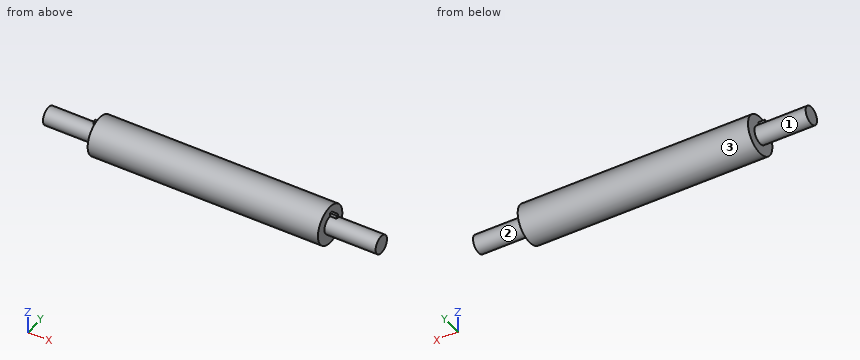
from build123d import *

# Parameters (mm, degrees)
BOSS_EXTRUDE1_START = 5
BOSS_EXTRUDE1_DEPTH = 5


with BuildPart() as part:
    # Sketch2 → Revolve1 (revolve)
    with BuildSketch(Plane.XY, mode=Mode.PRIVATE) as revolve1_sk:
        Polygon((130, 0), (-130, 0), (-130, -7), (-90, -7), (-90, -15), (90, -15), (90, -7), (130, -7), align=None)
    revolve(revolve1_sk.sketch.rotate(Axis((130, 0, 0), (-1, 0, 0)), 180), axis=Axis((130, 0, 0), (-1, 0, 0)))

    # Sketch3 → Boss-Extrude1 (add)
    with BuildSketch(Plane(origin=(90, 0, 0), x_dir=(0, 0, -1), z_dir=(1, 0, 0)).offset(BOSS_EXTRUDE1_START)):
        with BuildLine():
            Line((-7, 0), (-9.611930855, 0))
            Line((-9.611930855, 0), (-9.611930855, 2.103316634))
            Line((-9.611930855, 2.103316634), (-6.676530471, 2.103316634))
            ThreePointArc((-6.676530471, 2.103316634), (-6.918660033, 1.064022251), (-7, 0))
        make_face()
    boss_extrude1 = extrude(amount=-BOSS_EXTRUDE1_DEPTH)

    # Mirror1: Boss-Extrude1 across plane
    add(boss_extrude1.mirror(Plane(origin=(0, 0, 0), x_dir=(0, 0, 1), z_dir=(1, 0, 0))))


solid = part.part
Work out the finished part from the listing and answer in its coordinate system (mm). Face numbers are marked on the shaded views. A direction names the side the tool comes from. Coordinates: 2 decimals unless noted, no trailing zeros. Loops run counter-clockwise (first coordinate to the right, second up) from the corner with the lowest first, then second, coordinate; pieces in that order, holes last. Notation, with made-up numbers: M 18,78 L 27,78 A20 ccw 27,99 Z; hole C 54.25,-25 d10. An arc over 180 degrees is marked long. Answer in a Markdown table with one row per item. Add a question column.
1. Find section B-B, the plane x = -114. Write down the section's boundary in (y, z), then the cut area to 3 significant figures.
2. Find section A-A, the plane z = 0. Write down the section's boundary in (x, y).
3. Flat-ended cylindrical pins translate along their axes: P1, Ø1, axis at x = -25, y = -5.5, coming from the -Z side; P2, Ø1.3, axis at x = 93.5, z = 8, coming from the -Y side; P3, Ø1.7, axis at y = 1.5, z = 9, coming from the -X side; P4, Ø5, axis at x = -18.5, z = -2.5, coming from the -Y side. Find the tip coordinate at first contact, or state that the pin passes through.
4. Find section C-C, the plane y = -2.5. Write down the section's boundary in (x, z).
5. Consider L1, parallel to X at y = -8.5, z = -2.5; L2, parallel to Y at x = 51.5, z = -0.5; L3, parallel to Z at x = -47.5, y = 1. Determine where each line is inside the solid, lowest interval first.
6. A tool of negligible diameter and unlimited length cuts with its end or side. For the marked faces 1, 2 and 3, from which of +Z, -Z, +X, -X, +Y, -Y can it reach the whole face along a straight path? Write none if from no direction.
7. Find section D-D, the plane x = 83.5. Write down the section's boundary in (y, z).
Reported:
| question | item | result |
|---|---|---|
| 1 | outline | C 0,0 d14 |
| 1 | area | 154 mm^2 |
| 2 | outline | M -130,-7 L -90,-7 L -90,-15 L 90,-15 L 90,-7 L 130,-7 L 130,7 L 90,7 L 90,15 L -90,15 L -90,7 L -130,7 Z |
| 3 | P1 | stops at z = -14.14 |
| 3 | P2 | stops at y = 0 |
| 3 | P3 | stops at x = -95 |
| 3 | P4 | stops at y = -15 |
| 4 | outline | M -130,-6.54 L -90,-6.54 L -90,-14.79 L 90,-14.79 L 90,-6.54 L 130,-6.54 L 130,6.54 L 90,6.54 L 90,14.79 L -90,14.79 L -90,6.54 L -130,6.54 Z |
| 5 | L1 | x = -90 to 90 |
| 5 | L2 | y = -14.99 to 14.99 |
| 5 | L3 | z = -14.97 to 14.97 |
| 6 | face 1 | -X |
| 6 | face 2 | +X |
| 6 | face 3 | +X, -X |
| 7 | outline | C 0,0 d30 |
